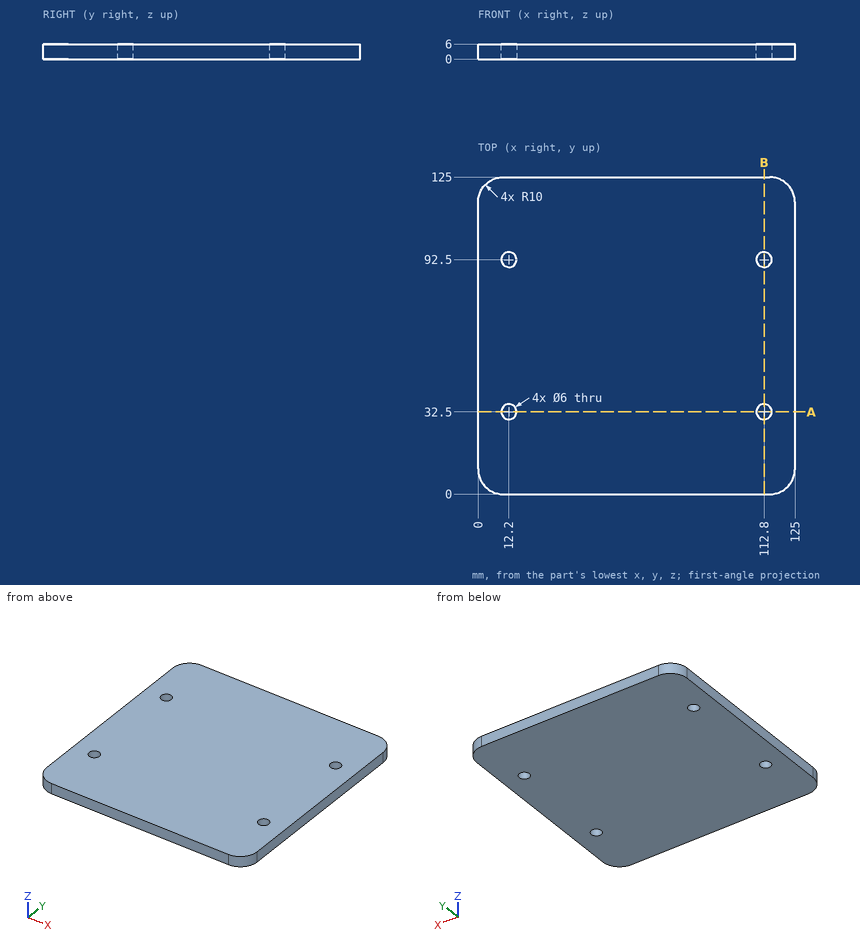
Study the drawing (mm; zero at the part's minimum x, y, z) and answer. Round coordinates to 2 decimals unless told otherwise and drop trailing zeros. Write each loop counter-clockwise with the first axis right and the second up, starting at its lowest first coordinate (ties: lowest second). Pieces come first, ordered by that corner, then holes.
1) A cutting plane is placed at A-A on y = 32.5. Determine the outline of the cut face in (x, z), and give its area (3 significant figures).
2) Consider probe 1 along Y at (x, z) = (12.2, 2.15); probe 2 along X at (y, z) = (93.5, 2.85); probe 3 along Y at (x, z) = (110.5, 1.1). Determine where each line is inside the solid, lowest interval first.
3) A flat-ended cylindrical pin translates along its axis: P1, Ø1.5, axis at y = 16.5, z = 1, coming from the -X side. Find the tip coordinate at first contact, or state that the pin passes through.
4) A cutting plane is placed at B-B on x = 112.8. Determine the outline of the cut face in (y, z), and give its area (3 significant figures).
Entries:
1. outline: (0, 0) - (9.2, 0) - (9.2, 6) - (0, 6) - close; (15.2, 0) - (109.8, 0) - (109.8, 6) - (15.2, 6) - close; (115.8, 0) - (125, 0) - (125, 6) - (115.8, 6) - close
1. area: 678 mm2
2. probe 1: y = 0 to 29.5, 35.5 to 89.5, 95.5 to 125
2. probe 2: x = 0 to 9.37, 15.03 to 109.97, 115.63 to 125
2. probe 3: y = 0 to 30.57, 34.43 to 90.57, 94.43 to 125
3. P1: stops at x = 0
4. outline: (0, 0) - (29.5, 0) - (29.5, 6) - (0, 6) - close; (35.5, 0) - (89.5, 0) - (89.5, 6) - (35.5, 6) - close; (95.5, 0) - (125, 0) - (125, 6) - (95.5, 6) - close
4. area: 678 mm2
